Here's the drawing with two shaded views (mm, measured from the low corner). I have some questions. A direction names the side the tool comes from. Coordinates: 2 decimals unless noted, no trailing zeros. Loops run counter-clockwise (first coordinate to the right, second up) from the corner with the lowest first, then second, coordinate; pieces in that order, holes last.
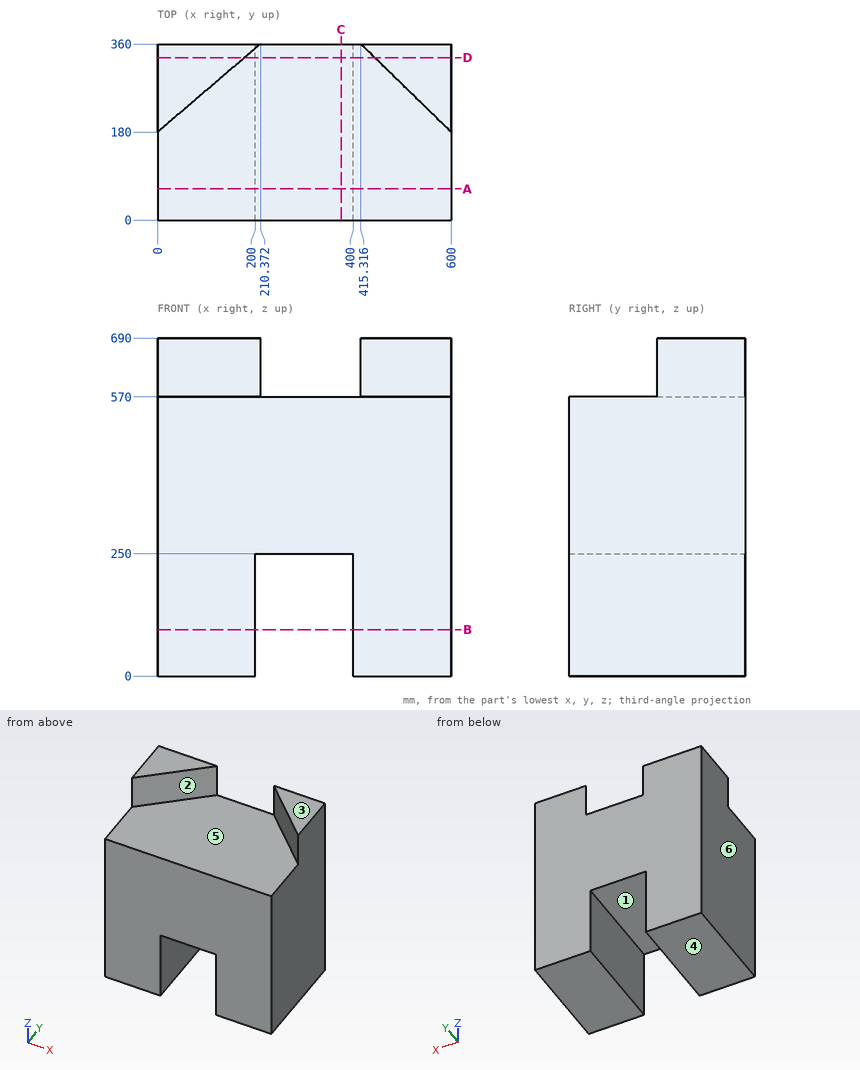
(1) If we mould it in two halves opening along X, with no side actions, what happens to the marked faces 4, 5 and 6? For each: released by +X, released by -X, zero draft, split by the parting line, or undercut.
Check values:
face 4: zero draft
face 5: undercut
face 6: released by -X
(2) I want a section at B-B on z = 94.5. Write out the boundary of the cut face in (x, y), then the cut area to 3 significant figures.
Check values:
outline: (0, 0) - (200, 0) - (200, 360) - (0, 360) - close; (400, 0) - (600, 0) - (600, 360) - (400, 360) - close
area: 144,000 mm2
(3) Which directions (+Z, -Z, +X, -X, +Y, -Y) give clear straight access to the entire face, cutting with the end or side of a thin tool? Please do the marked faces 1, 2 and 3.
Check values:
face 1: -Z, +Y, -Y
face 2: +Z, -Y
face 3: +Z, +X, -X, +Y, -Y
(4) If I drill on probe 1 along X at (y, z) = (142, 193.5); probe 2 along Z at (x, y) = (154.5, 55.5); probe 3 along X at (y, z) = (334, 612) (1 decimal), over which ranges is the centre line in solid material (lowest first)?
Check values:
probe 1: x = 0 to 200, 400 to 600
probe 2: z = 0 to 570
probe 3: x = 0 to 180, 442 to 600
(5) I want a section at A-A on y = 64. Write out the boundary of the cut face in (x, z), then the cut area to 3 significant figures.
Check values:
outline: (0, 0) - (200, 0) - (200, 250) - (400, 250) - (400, 0) - (600, 0) - (600, 570) - (0, 570) - close
area: 292,000 mm2
(6) I want a section at C-C on x = 375. Write out the boundary of the cut face in (y, z).
Check values:
outline: (0, 250) - (360, 250) - (360, 570) - (0, 570) - close
(7) I want a section at D-D on y = 332. Write out the boundary of the cut face in (x, z) (1 decimal), then the cut area to 3 significant figures.
Check values:
outline: (0, 0) - (200, 0) - (200, 250) - (400, 250) - (400, 0) - (600, 0) - (600, 690) - (444, 690) - (444, 570) - (177.6, 570) - (177.6, 690) - (0, 690) - close
area: 332,000 mm2
(8) I'm going to push flat-ended pins straight in: pin 1 (2 mm diameter, centred on x = 327.5, z = 460, fed in from -Y); pin 2 (10 mm diameter, centred on x = 217, y = 40, fed in from +Z). Where does each tip first touch, or does it pass through?
Check values:
pin 1: stops at y = 0
pin 2: stops at z = 570
